from build123d import *

# Parameters (mm, degrees)
F0_W      = 127
F0_H      = 76.2
F1_DEPTH  = 3.175
F2_R      = 1.5875
F2_W      = 12.7
F2_H      = 12.7
F2_W_2    = 9.525
F2_H_2    = 9.525
F2_W_3    = 6.35
F2_H_3    = 6.35
F2_W_4    = 3.175
F2_H_4    = 3.175
F3_DEPTH  = 3.175
F4_W      = 25.4
F4_H      = 25.4
F4_W_2    = 12.7
F4_H_2    = 12.7
F4_W_3    = 6.35
F4_H_3    = 6.35
F4_W_4    = 3.175
F4_H_4    = 3.175
F5_DEPTH  = 6.35
F6_R      = 9.525
F6_R_2    = 3.175
F6_R_3    = 1.5875
F7_DEPTH  = 6.35
F8_R      = 12.7
F8_R_2    = 6.35
F8_R_3    = 9.525
F8_R_4    = 3.175
F8_R_5    = 1.5875
F9_DEPTH  = 6.35
F10_W     = 3.175
F10_H     = 3.175
F11_DEPTH = 6.35
F12_W     = 76.2
F12_H     = 5.08
F13_DEPTH = 6.35
F15_DEPTH = 5.08
F16_R     = 6.35
F18_DEPTH = 3.175
F19_W     = 25.4
F19_H     = 19.05
F20_DEPTH = 3.175


with BuildPart() as f1:
    # F0 (on Top) → F1 (new body)
    with BuildSketch(Plane.XY):
        Rectangle(F0_W, F0_H)
    extrude(amount=F1_DEPTH)

    # F2 (on face) → F3 (cut, through all)
    with BuildSketch(Plane.XY.offset(3.175)):
        with BuildLine():
            ThreePointArc((-44.499805, 26.19375), (-57.137537, 25.002345), (-44.45, 25.4))
            ThreePointArc((-44.45, 25.4), (-44.462463, 25.797655), (-44.499805, 26.19375))
        make_face()
        with BuildLine():
            ThreePointArc((-22.449121, 28.971875), (-25.996094, 31.725098), (-28.749316, 28.178125))
            Line((-28.749316, 28.178125), (-22.449121, 28.971875))
        make_face()
        with BuildLine():
            Line((-22.449121, 28.971875), (-28.749316, 28.178125))
            ThreePointArc((-28.749316, 28.178125), (-25.400391, 25.406232), (-22.424219, 28.575))
            ThreePointArc((-22.424219, 28.575), (-22.43045, 28.773828), (-22.449121, 28.971875))
        make_face()
        with BuildLine():
            ThreePointArc((-33.474463, 27.582813), (-38.794922, 31.712646), (-42.924756, 26.392188))
            Line((-42.924756, 26.392188), (-33.474463, 27.582813))
        make_face()
        with BuildLine():
            Line((-33.474463, 27.582813), (-42.924756, 26.392188))
            ThreePointArc((-42.924756, 26.392188), (-37.901368, 22.234348), (-33.437109, 26.9875))
            ThreePointArc((-33.437109, 26.9875), (-33.446457, 27.285742), (-33.474463, 27.582813))
        make_face()
        with Locations((-12.998828, 30.1625)):
            Circle(F2_R)
        with Locations((50.8, 25.4)):
            Rectangle(F2_W, F2_H)
        with Locations((33.3375, 23.8125)):
            Rectangle(F2_W_2, F2_H_2)
        with Locations((19.05, 22.225)):
            Rectangle(F2_W_3, F2_H_3)
        with Locations((7.9375, 20.6375)):
            Rectangle(F2_W_4, F2_H_4)
    extrude(amount=-F3_DEPTH, mode=Mode.SUBTRACT)

    # F4 (on face) → F5 (join)
    with BuildSketch(Plane.XY.offset(3.175)):
        with Locations((-41.275, -15.875)):
            Rectangle(F4_W, F4_H)
        with Locations((-12.7, -9.525)):
            Rectangle(F4_W_2, F4_H_2)
        with Locations((6.35, -6.35)):
            Rectangle(F4_W_3, F4_H_3)
        with Locations((20.6375, -4.7625)):
            Rectangle(F4_W_4, F4_H_4)
    extrude(amount=F5_DEPTH)

    # F6 (on face) → F7 (cut)
    with BuildSketch(Plane.XY.offset(9.525)):
        with Locations((-41.275, -15.875)):
            Circle(F6_R)
        with Locations((-12.7, -9.525)):
            Circle(F6_R_2)
        with Locations((6.35, -6.35)):
            Circle(F6_R_3)
    extrude(amount=-F7_DEPTH, mode=Mode.SUBTRACT)

    # F8 (on face) → F9 (join)
    with BuildSketch(Plane.XY.offset(3.175)):
        with Locations((47.625, -22.225)):
            Circle(F8_R)
        with Locations((-6.35, -28.575)):
            Circle(F8_R_2)
        with Locations((15.875, -25.4)):
            Circle(F8_R_3)
        with Locations((57.15, 3.175)):
            Circle(F8_R_4)
        with Locations((-20.6375, -33.3375)):
            Circle(F8_R_5)
    extrude(amount=F9_DEPTH)

    # F10 (on face) → F11 (cut)
    with BuildSketch(Plane.XY.offset(9.525)):
        Polygon((52.3875, -17.4625), (42.8625, -17.4625), (42.8625, -26.9875), align=None)
        Polygon((52.3875, -26.9875), (52.3875, -17.4625), (42.8625, -26.9875), align=None)
        Polygon((20.6375, -20.6375), (11.1125, -20.6375), (11.1125, -30.1625), align=None)
        Polygon((20.6375, -30.1625), (20.6375, -20.6375), (11.1125, -30.1625), align=None)
        with Locations((-6.35, -28.575)):
            Rectangle(F10_W, F10_H)
    extrude(amount=-F11_DEPTH, mode=Mode.SUBTRACT)

    # F12 (on face) → F13 (join)
    with BuildSketch(Plane.XY.offset(3.175)):
        with Locations((-19.05, 10.16)):
            Rectangle(F12_W, F12_H)
    extrude(amount=F13_DEPTH)

    # F14 (on face) → F15 (cut, through all)
    with BuildSketch(Plane(origin=(0, 12.7, 0), x_dir=(-1, 0, 0), z_dir=(0, 1, 0))):
        Polygon((53.483826, 9.525), (57.15, 3.175), (57.15, 9.525), align=None)
        Polygon((45.863826, 3.175), (53.483826, 3.175), (49.817652, 9.525), (40.535543, 9.525), align=None)
        Polygon((34.099158, 3.175), (41.719158, 3.175), (36.390875, 9.525), (27.749158, 9.525), align=None)
        Polygon((14.421394, 9.525), (21.98903, 3.175), (29.60903, 3.175), (23.25903, 9.525), align=None)
        Polygon((-1.701477, 3.175), (17.049606, 3.175), (9.481971, 9.525), (-12.7, 9.525), align=None)
        Polygon((-19.05, 3.175), (-8.051477, 3.175), (-19.05, 9.525), align=None)
    extrude(amount=-F15_DEPTH, mode=Mode.SUBTRACT)

    # F16
    f16_edges = [f1.edges().sort_by_distance(p)[0] for p in [
        (63.5, -38.1, 1.5875),
        (-63.5, -38.1, 1.5875),
        (-63.5, 38.1, 1.5875),
        (63.5, 38.1, 1.5875),
    ]]
    fillet(f16_edges, radius=F16_R)

    # F17 (on face) → F18 (cut, through all)
    with BuildSketch(Plane.XY.offset(3.175)):
        Polygon((-9.660837, 15.875), (16.63156, 30.48), (25.4, 30.48), (25.4, 35.56), (12.7, 35.56), (-17.021839, 19.05), (-38.1, 19.05), (-38.1, 15.875), align=None)
    extrude(amount=-F18_DEPTH, mode=Mode.SUBTRACT)

    # F19 (on face) → F20 (cut, through all)
    with BuildSketch(Plane.XY.offset(3.175)):
        with Locations((38.1, 4.445)):
            Rectangle(F19_W, F19_H)
    extrude(amount=-F20_DEPTH, mode=Mode.SUBTRACT)


solid = f1.part
Geometry: final body of the model. Coordinates: model frame, mm. A direction names the side the tool comes from. Round coordinates to 2 decimals unless told otherwise and drop trailing zeros. Loops run counter-clockwise (first coordinate to the right, second up) from the corner with the lowest first, then second, coordinate; pieces in that order, holes last. Notation, with made-up numbers: M -38,36 L 4,36 A23 ccw 4,62 Z; hole C 5.5,49.5 d4. An arc over 180 degrees is marked long. Put each result on its own line as item: value. Start each with the question number.
(1) Material intervals for line 1 along X through (y, z) = (-4, 7) (3 decimals); line 2 along Y through (x, z) = (18, 2); line 3 along X through (y, z) = (-6, 8) (3 decimals), sorted ascending. Write a range as [from, to].
(2) Contact query for flat-ended pins moving along their axis: pin 1 Ø3 at (y, z) = (-5.5, 6) entering from -X (3 decimals); pin 2 Ø1.9 at (x, z) = (-55, 6.5) entering from +Y; pin 3 Ø1.6 at (x, z) = (-7, 5) entering from -Y (3 decimals). Output: stop coordinate, or through.
(3) Section query A-A (z = 7). State how many separate pieces and enclosed holes the cut face has, then the cut area to 3 significant figures.
(4) Draft query along X for faces 1 (the face through (-1, 1, 0)), 2 (the face through (61.59, 36.29, 1.61)), 3 (the face through (9.525, 21, 2)). Return one class per face: +X half, -X half, draft (parallel to the pull), parting line (faces both ways), or undercut.
(5) Section query B-B (y = -14). Return loops of the section in (x, z) (3 decimals), then the cut area to 3 significant figures.
(6) Set-up query: faces 4 (the face through (10, 12.7, 6)), 5 (the face through (-21.808, -32.265, 6.306)), 6 (the face through (57.15, 25, 2)). Return all of +Z, -Z, +X, -X, +Y, -Y with unobstructed straight access to the full face (end or side cutting, diameter ignored); none if empty.
Findings below:
1. line 1: x = [-53.975, -28.575], [-19.05, -6.35], [3.175, 9.525], [19.05, 22.225]
1. line 2: y = [-38.1, 19.05], [25.4, 30.48], [35.56, 38.1]
1. line 3: x = [-53.975, -28.575], [-19.05, -6.35], [3.175, 4.802], [7.898, 9.525], [19.05, 22.225]
2. pin 1: stops at x = -53.975
2. pin 2: stops at y = 12.7
2. pin 3: stops at y = -34.925
3. separate pieces: 14
3. enclosed holes: 6
3. area: 1,420 mm2
4. face 1: draft
4. face 2: +X half
4. face 3: undercut
5. outline: M -63.5,0 L 63.5,0 L 63.5,3.175 L 57.302,3.175 L 57.302,9.525 L 37.948,9.525 L 37.948,3.175 L -6.35,3.175 L -6.35,9.525 L -19.05,9.525 L -19.05,3.175 L -28.575,3.175 L -28.575,9.525 L -31.936,9.525 L -31.936,3.175 L -50.614,3.175 L -50.614,9.525 L -53.975,9.525 L -53.975,3.175 L -63.5,3.175 Z
5. area: 649 mm2
6. face 4: +Z, +X, -X, +Y
6. face 5: +Z
6. face 6: +Z, -Z
